CAD build for the part. Positions are in the model's coordinates, mm. Coordinates: 2 decimals unless noted, no trailing zeros. Loops run counter-clockwise (first coordinate to the right, second up) from the corner with the lowest first, then second, coordinate; pieces in that order, holes last. Notation, with made-up numbers: (50, 17) -> (80, 17) arc R14 cw to (80, 27) -> close; hole circle Ø8 at (50.5, 33). An arc over 180 degrees is marked (long way). Write item = value, one per line. Start each with the question number.
(1) Flat gauge pins, fed straight in: P1, Ø24, axis at x = -48, z = -1, coming from the +Y side; P2, Ø11, axis at x = 42, z = -1, coming from the +Y side; P3, Ø3, axis at y = 6.5, z = 4, coming from the -X side. Where does each tip first touch, or does it go through?
(2) Band-saw the part on D-D (x = 45). Write the cut outline in (y, z), and give its area (3 significant figures).
(3) Drill centre lines: line 1 (X direction, y = 2, z = 0); line 2 (X direction, y = 4, z = 0); line 3 (Y direction, x = 39, z = 6.5). Where is each one in solid material? Low to high. Write a range as from..to.
(4) Band-saw the part on A-A (y = 7.25). Write the cut outline in (x, z).
(5) Band-saw the part on B-B (x = 0). Write the cut outline in (y, z), and give its area (3 significant figures).
(6) Band-saw the part on C-C (z = 9). Write the cut outline in (x, y), and give its area (3 significant figures).
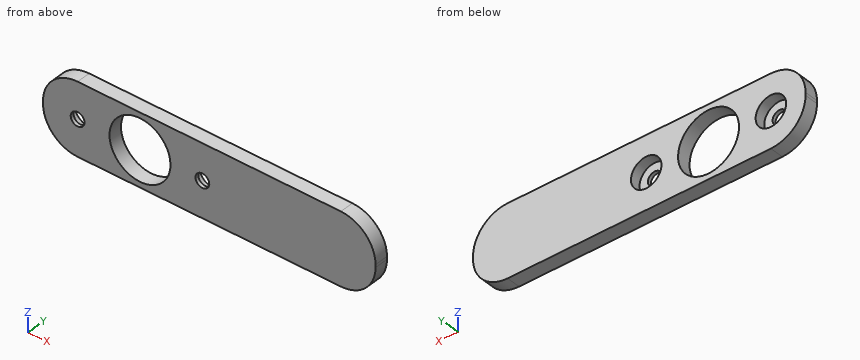
```python
from build123d import *

# Parameters (mm, degrees)
SKETCH1_R           = 11
SKETCH1_R_2         = 22
BOSS_EXTRUDE1_DEPTH = 10
BOSS_EXTRUDE4_DEPTH = 10
CUT_EXTRUDE1_DEPTH  = 10
BOSS_EXTRUDE5_DEPTH = 10
BOSS_EXTRUDE6_DEPTH = 10
SKETCH2_R           = 12.791308891
SKETCH2_R_2         = 5
SKETCH2_R_3         = 12.648974484
BOSS_EXTRUDE2_DEPTH = 2.5
CUT_EXTRUDE2_DEPTH  = 10
FILLET1_R           = 25
BOSS_EXTRUDE7_DEPTH = 10
FILLET2_R           = 25
FILLET3_R           = 25
CUT_EXTRUDE5_DEPTH  = 10
BOSS_EXTRUDE8_DEPTH = 10
BOSS_EXTRUDE9_DEPTH = 10
FILLET4_R           = 25


with BuildPart() as part:
    # Sketch1 → Boss-Extrude1 (new body)
    with BuildSketch(Plane(origin=(0, 0, 0), x_dir=(1, 0, 0), z_dir=(0, 1, 0))):
        with BuildLine():
            Line((-70, -27), (-25, -27))
            Line((-25, -27), (25, -27))
            Line((25, -27), (70, -27))
            Line((70, -27), (70, 0))
            ThreePointArc((70, 0), (62.67766953, 17.67766953), (45, 25))
            Line((45, 25), (-45, 25))
            ThreePointArc((-45, 25), (-62.67766953, 17.67766953), (-70, 0))
            Line((-70, 0), (-70, -27))
        make_face()
        with Locations(Location((-45, 0, 0), (0, 0, 90))):  # turned: the seam where the file's is
            Circle(SKETCH1_R, mode=Mode.SUBTRACT)
        with Locations(Location((0, 0, 0), (0, 0, 270))):  # turned: the seam where the file's is
            Circle(SKETCH1_R_2, mode=Mode.SUBTRACT)
        with Locations(Location((45, 0, 0), (0, 0, 270))):  # turned: the seam where the file's is
            Circle(SKETCH1_R, mode=Mode.SUBTRACT)
    extrude(amount=BOSS_EXTRUDE1_DEPTH)

    # Sketch3_2 → Boss-Extrude4 (add)
    with BuildSketch(Plane(origin=(0, 10, 0), x_dir=(1, 0, 0), z_dir=(0, 1, 0))):
        Polygon((-70, -27), (-121.413521395, -27), (-121.413521395, 25), (-45, 25), (-60.069243324, 8.259929081), align=None)
    extrude(amount=-BOSS_EXTRUDE4_DEPTH)

    # Sketch3 → Cut-Extrude1 (cut)
    with BuildSketch(Plane(origin=(0, 10, 0), x_dir=(1, 0, 0), z_dir=(0, 1, 0))):
        Polygon((-70, -27), (-121.413521395, -27), (-121.413521395, 25), (-45, 25), (-60.069243324, 8.259929081), align=None)
    extrude(amount=-CUT_EXTRUDE1_DEPTH, mode=Mode.SUBTRACT)

    # Sketch5 → Boss-Extrude5 (add)
    with BuildSketch(Plane(origin=(0, 10, 0), x_dir=(1, 0, 0), z_dir=(0, 1, 0))):
        Polygon((-70, -27), (-152.396081637, -27), (-152.396081637, 25), (-45, 25), (-47.056495807, 18.199026423), (-57.650043642, 5.920141433), (-62.706055109, -17.674578746), align=None)
    extrude(amount=-BOSS_EXTRUDE5_DEPTH)

    # Sketch6 → Boss-Extrude6 (add)
    with BuildSketch(Plane(origin=(0, 10, 0), x_dir=(1, 0, 0), z_dir=(0, 1, 0))):
        Polygon((-170, -27), (-147.259885351, -27), (-136.049250897, -7.734745997), (-143.609911342, 12.600823478), (-152.396081637, 25), (-170, 25), align=None)
    extrude(amount=-BOSS_EXTRUDE6_DEPTH)

    # Sketch2 → Boss-Extrude2 (add)
    with BuildSketch(Plane.XZ):
        with Locations((-45, 0)):
            Circle(SKETCH2_R)
        with Locations(Location((-45, 0, 0), (0, 0, 270))):  # turned: the seam where the file's is
            Circle(SKETCH2_R_2, mode=Mode.SUBTRACT)
        with Locations((45, 0)):
            Circle(SKETCH2_R_3)
        with Locations(Location((45, 0, 0), (0, 0, 270))):  # turned: the seam where the file's is
            Circle(SKETCH2_R_2, mode=Mode.SUBTRACT)
    extrude(amount=-BOSS_EXTRUDE2_DEPTH)

    # Sketch7 → Cut-Extrude2 (cut)
    with BuildSketch(Plane(origin=(0, 10, 0), x_dir=(1, 0, 0), z_dir=(0, 1, 0))):
        Polygon((-70, -27), (-70, 25), (-80.950376598, 84.263900648), (-214.684311222, 75.641343309), (-217.522149123, -21.969417176), (-150.276663253, -84.577260073), align=None)
    extrude(amount=-CUT_EXTRUDE2_DEPTH, mode=Mode.SUBTRACT)

    # Fillet1
    fillet1_edges = [part.edges().sort_by_distance(p)[0] for p in [
        (-70, 5, -25),
    ]]
    fillet(fillet1_edges, radius=FILLET1_R)

    # Sketch8 → Boss-Extrude7 (add)
    with BuildSketch(Plane(origin=(0, 10, 0), x_dir=(1, 0, 0), z_dir=(0, 1, 0))):
        Polygon((45, 25), (170, 25), (170, -27), (70, -27), (59.971259961, 0), align=None)
    extrude(amount=-BOSS_EXTRUDE7_DEPTH)

    # Fillet2
    fillet2_edges = [part.edges().sort_by_distance(p)[0] for p in [
        (170, 5, -25),
    ]]
    fillet(fillet2_edges, radius=FILLET2_R)

    # Fillet3
    fillet3_edges = [part.edges().sort_by_distance(p)[0] for p in [
        (-70, 5, 27),
        (170, 5, 27),
    ]]
    fillet(fillet3_edges, radius=FILLET3_R)

    # Sketch9 → Cut-Extrude5 (cut)
    with BuildSketch(Plane(origin=(0, 10, 0), x_dir=(1, 0, 0), z_dir=(0, 1, 0))):
        with BuildLine():
            Line((168.265391903, -53.084180291), (170, -26))
            Line((170, -26), (152, -26))
            ThreePointArc((152, -26), (148.535533906, -26.748737342), (145, -27))
            Line((145, -27), (-45, -27))
            ThreePointArc((-45, -27), (-48.535533906, -26.748737342), (-52, -26))
            Line((-52, -26), (-70, -26))
            Line((-70, -26), (-6.059888958, -84.123320181))
            Line((-6.059888958, -84.123320181), (168.265391903, -53.084180291))
        make_face()
        with BuildLine():
            ThreePointArc((145, -27), (148.535533906, -26.748737342), (152, -26))
            Line((152, -26), (-52, -26))
            ThreePointArc((-52, -26), (-48.535533906, -26.748737342), (-45, -27))
            Line((-45, -27), (145, -27))
        make_face()
    extrude(amount=-CUT_EXTRUDE5_DEPTH, mode=Mode.SUBTRACT)

    # Sketch10 → Boss-Extrude8 (add)
    with BuildSketch(Plane(origin=(0, 10, 0), x_dir=(1, 0, 0), z_dir=(0, 1, 0))):
        with BuildLine():
            Line((-14.39135104, -23.974647324), (-57.930920378, -15.319190769))
            Line((-57.930920378, -15.319190769), (-70, 0))
            Line((-70, 0), (-70, -2))
            ThreePointArc((-70, -2), (-65, -17), (-52, -26))
            Line((-52, -26), (152, -26))
            ThreePointArc((152, -26), (165, -17), (170, -2))
            Line((170, -2), (170, 0))
            Line((170, 0), (125.93195978, -21.351781701))
            Line((125.93195978, -21.351781701), (-14.39135104, -23.974647324))
        make_face()
        with BuildLine():
            Line((170, -26), (170, -2))
            ThreePointArc((170, -2), (165, -17), (152, -26))
            Line((152, -26), (170, -26))
        make_face()
        with BuildLine():
            ThreePointArc((-52, -26), (-65, -17), (-70, -2))
            Line((-70, -2), (-70, -26))
            Line((-70, -26), (-52, -26))
        make_face()
    extrude(amount=-BOSS_EXTRUDE8_DEPTH)

    # Sketch11 → Boss-Extrude9 (add)
    with BuildSketch(Plane(origin=(0, 10, 0), x_dir=(1, 0, 0), z_dir=(0, 1, 0))):
        with BuildLine():
            Line((-57.382853391, 13.015294561), (-70, 0))
            ThreePointArc((-70, 0), (-62.67766953, 17.67766953), (-45, 25))
            Line((-45, 25), (145, 25))
            ThreePointArc((145, 25), (162.67766953, 17.67766953), (170, 0))
            Line((170, 0), (115.178210727, 18.515775765))
            Line((115.178210727, 18.515775765), (14.984743936, 21.925501075))
            Line((14.984743936, 21.925501075), (-3.225773035, 23.26883074))
            Line((-3.225773035, 23.26883074), (-31.681488845, 16.787813616))
            Line((-31.681488845, 16.787813616), (-57.382853391, 13.015294561))
        make_face()
        with BuildLine():
            Line((170, 0), (170, 26))
            Line((170, 26), (-70, 26))
            Line((-70, 26), (-70, 0))
            ThreePointArc((-70, 0), (-62.67766953, 17.67766953), (-45, 25))
            Line((-45, 25), (145, 25))
            ThreePointArc((145, 25), (162.67766953, 17.67766953), (170, 0))
        make_face()
    extrude(amount=-BOSS_EXTRUDE9_DEPTH)

    # Fillet4
    fillet4_edges = [part.edges().sort_by_distance(p)[0] for p in [
        (170, 5, 26),
        (-70, 5, 26),
        (-70, 5, -26),
        (170, 5, -26),
    ]]
    fillet(fillet4_edges, radius=FILLET4_R)


solid = part.part
```
Findings below:
q1.P1 = 10
q1.P2 = 2.5
q1.P3 = -69.95
q2.outline = (0, -26) -> (10, -26) -> (10, -11) -> (2.5, -11) -> (2.5, -5) -> (0, -5) -> close; (0, 5) -> (2.5, 5) -> (2.5, 11) -> (10, 11) -> (10, 26) -> (0, 26) -> close
q2.area = 330 mm²
q3.line_1 = -70..-50, -40..-22, 22..40, 50..170
q3.line_2 = -70..-56, -34..-22, 22..34, 56..170
q3.line_3 = 0..2.5
q4.outline = (-70, -1) arc R25 ccw to (-45, -26) -> (145, -26) arc R25 ccw to (170, -1) -> (170, 1) arc R25 ccw to (145, 26) -> (-45, 26) arc R25 ccw to (-70, 1) -> close; hole circle Ø22 at (-45, 0); hole circle Ø44 at (0, 0); hole circle Ø22 at (45, 0)
q5.outline = (0, -26) -> (10, -26) -> (10, -22) -> (0, -22) -> close; (0, 22) -> (10, 22) -> (10, 26) -> (0, 26) -> close
q5.area = 80.0 mm²
q6.outline = (-68.69, 0) -> (-20.07, 0) -> (-20.07, 10) -> (-38.68, 10) -> (-38.68, 2.5) -> (-51.32, 2.5) -> (-51.32, 10) -> (-68.69, 10) -> close; (20.07, 0) -> (168.69, 0) -> (168.69, 10) -> (51.32, 10) -> (51.32, 2.5) -> (38.68, 2.5) -> (38.68, 10) -> (20.07, 10) -> close
q6.area = 1,780 mm²
